Source: CAD feature listing. Evaluate the final solid. Frame: model axes, mm. Face numbers are marked on the shaded views. A direction names the side the tool comes from. Round coordinates to 2 decimals unless told otherwise and drop trailing zeros. Order: outer loops, then holes, each group sorted by start corner. A loop starts at its lowest first (then second) coordinate and runs counter-clockwise, first axis right, second up. Notation, with made-up numbers: (87.5, 4.25) - (123.5, 4.25) arc R34 cw to (123.5, 40.25) - close; hole circle Ø3 at (-38, 86). An arc over 180 degrees is marked (long way). Use one line per item in the form item = value. Start each with the question number.
Q1. Pin query (flat end, axial travel): pin 1 Ø7.5 at (y, z) = (41, 9) entering from +X; pin 2 Ø10.5 at (x, z) = (-64, 9) entering from -Y; pin 3 Ø2 at (x, z) = (109.5, 12) entering from +Y; pin 4 Ø1.5 at (x, y) = (88.5, 2.5) entering from +Z. Return the tip coordinate at first contact, or that it passes through.
Q2. Draft query along Y for the marked faces 1, 2 and 3. Return one class per face: released by +Y, released by -Y, zero draft, split by the parting line, or undercut.
Q3. Cut plane D-D, the plane y = 100.5. Return the cut outline in (x, z).
Q4. Set-up query: the marked faces 4, 5 and 6. Return all of +Z, -Z, +X, -X, +Y, -Y with unobstructed straight access to the full face (end or side cutting, diameter ignored); none if empty.
Q5. Ray query, line 1 (X direction, y = 28, z = 18.25); line 2 (Y direction, x = 24, z = 10); line 3 (X direction, y = -69, z = 5). Return the intervals inside material, ascending. Write a range as [from, to].
Q6. Cut plane B-B, the plane x = 25.5. Return the cut outline in (y, z), and give its area (3 significant figures).
Q7. Cut plane C-C, the plane y = 39. Return the cut outline in (x, z).
Q8. Cut plane A-A, the plane z = 5.5. Return the cut outline in (x, y).
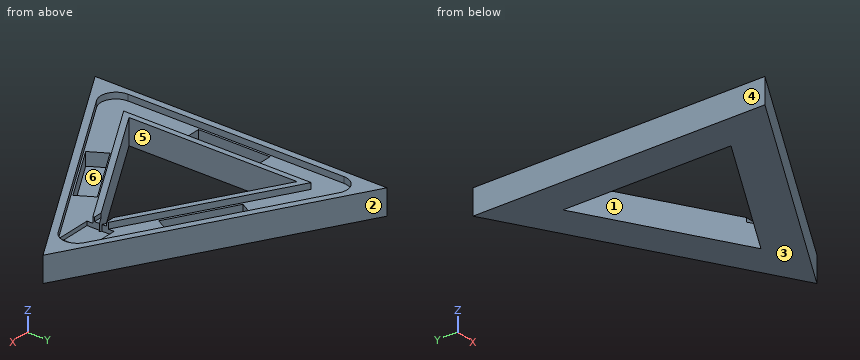
from build123d import *

# Parameters (mm, degrees)
PRISM003_DEPTH         = 6
PRISM002_DEPTH         = 6
BOX004_W               = 10
BOX004_H               = 12
BOX004_DEPTH           = 4
BOX003_W               = 35
BOX003_H               = 26.5
BOX003_DEPTH           = 10
BOX002_W               = 70
BOX002_H               = 19
BOX002_DEPTH           = 19
BOX002_PLACEMENT_ANGLE = 30
BOX001_W               = 70
BOX001_H               = 19
BOX001_DEPTH           = 19
BOX001_PLACEMENT_ANGLE = 90
BOX_W                  = 70
BOX_H                  = 19
BOX_DEPTH              = 19
BOX_PLACEMENT_ANGLE    = 30
PRISM001_DEPTH         = 25
PRISM_DEPTH            = 25
FILLET_R               = 15


with BuildPart() as prism003:
    # Prism003 → Prism003 (new body)
    with BuildSketch(Plane.XY.offset(13)):
        Polygon((106, 0), (-53, 91.798693), (-53, -91.798693), align=None)
    extrude(amount=PRISM003_DEPTH)


with BuildPart() as cut006:
    # Prism002 → Prism002 (new body)
    with BuildSketch(Plane.XY.offset(13)):
        Polygon((152, 0), (-76, 131.635861), (-76, -131.635861), align=None)
    extrude(amount=PRISM002_DEPTH)

    # Cut006: cut Prism003
    add(prism003.part, mode=Mode.SUBTRACT)


with BuildPart() as box004:
    # Box004 → Box004 (new body)
    with BuildSketch(Plane(origin=(84, -6, 15), x_dir=(1, 0, 0), z_dir=(0, 0, 1))):
        with Locations((5, 6)):
            Rectangle(BOX004_W, BOX004_H)
    extrude(amount=BOX004_DEPTH)


with BuildPart() as box003:
    # Box003 → Box003 (new body)
    with BuildSketch(Plane(origin=(93, -13.3, 9), x_dir=(1, 0, 0), z_dir=(0, 0, 1))):
        with Locations((17.5, 13.25)):
            Rectangle(BOX003_W, BOX003_H)
    extrude(amount=BOX003_DEPTH)


with BuildPart() as box002:
    # Box002 → Box002 (new body)
    with BuildSketch(Plane.XY):
        with Locations((35, 9.5)):
            Rectangle(BOX002_W, BOX002_H)
    extrude(amount=BOX002_DEPTH)


with BuildPart() as box002_1:
    # Box002 placement: moved
    add(box002.part.moved(Location((7, -82, 0))).rotate(Axis((7, -82, 0), (0, 0, 1)), BOX002_PLACEMENT_ANGLE))


with BuildPart() as box001:
    # Box001 → Box001 (new body)
    with BuildSketch(Plane.XY):
        with Locations((35, 9.5)):
            Rectangle(BOX001_W, BOX001_H)
    extrude(amount=BOX001_DEPTH)


with BuildPart() as box001_1:
    # Box001 placement: moved
    add(box001.part.moved(Location((-55, -35, 0))).rotate(Axis((-55, -35, 0), (0, 0, 1)), BOX001_PLACEMENT_ANGLE))


with BuildPart() as box:
    # Box → Box (new body)
    with BuildSketch(Plane.XY):
        with Locations((35, 9.5)):
            Rectangle(BOX_W, BOX_H)
    extrude(amount=BOX_DEPTH)


with BuildPart() as box_1:
    # Box placement: moved
    add(box.part.moved(Location((-2, 65, 0))).rotate(Axis((-2, 65, 0), (0, 0, -1)), BOX_PLACEMENT_ANGLE))


with BuildPart() as prism001:
    # Prism001 → Prism001 (new body)
    with BuildSketch(Plane.XY.offset(-6)):
        Polygon((95, 0), (-47.5, 82.272413), (-47.5, -82.272413), align=None)
    extrude(amount=PRISM001_DEPTH)


with BuildPart() as base_fillet:
    # Prism → Prism (new body)
    with BuildSketch(Plane.XY.offset(-6)):
        Polygon((165, 0), (-82.5, 142.894192), (-82.5, -142.894192), align=None)
    extrude(amount=PRISM_DEPTH)

    # Cut: cut Prism001
    add(prism001.part, mode=Mode.SUBTRACT)

    # Cut001: cut Box
    add(box_1.part, mode=Mode.SUBTRACT)

    # Cut002: cut Box001
    add(box001_1.part, mode=Mode.SUBTRACT)

    # Cut003: cut Box002
    add(box002_1.part, mode=Mode.SUBTRACT)

    # Cut004: cut Box003
    add(box003.part, mode=Mode.SUBTRACT)

    # Cut005: cut Box004
    add(box004.part, mode=Mode.SUBTRACT)

    # Cut007: cut Cut006
    add(cut006.part, mode=Mode.SUBTRACT)

    # Fillet
    fillet_edges = [base_fillet.edges().sort_by_distance(p)[0] for p in [
        (152, 0, 16),
        (-76, 131.635861, 16),
        (-76, -131.635861, 16),
    ]]
    fillet(fillet_edges, radius=FILLET_R)


solid = base_fillet.part
Completed:
q1.pin_1 = 100.48
q1.pin_2 = -135.24
q1.pin_3 = 32.62
q1.pin_4 = through
q2.face_1 = undercut
q2.face_2 = released by +Y
q2.face_3 = zero draft
q3.outline = (-82.5, -6) - (-9.07, -6) - (-9.07, 19) - (-22.07, 19) - (-22.07, 13) - (-76, 13) - (-76, 19) - (-82.5, 19) - close
q4.face_4 = +Z, -Z, -X, +Y, -Y
q4.face_5 = +Z, -Z
q4.face_6 = +Z
q5.line_1 = [-82.5, -76], [-53, -47.5], [46.5, 57.5], [103.5, 116.5]
q5.line_2 = [-81.41, -72.19], [-50.25, -40.99], [40.99, 49.99], [71.93, 81.41]
q5.line_3 = [-82.5, -47.5], [-24.51, -0.51], [29.52, 45.49]
q6.outline = (-80.54, -6) - (-40.13, -6) - (-40.13, 19) - (-46.48, 19) - (-46.48, 13) - (-49.38, 13) - (-49.38, 0) - (-71.32, 0) - (-71.32, 13) - (-73.03, 13) - (-73.03, 19) - (-80.54, 19) - close; (40.13, -6) - (80.54, -6) - (80.54, 19) - (73.03, 19) - (73.03, 13) - (71.06, 13) - (71.06, 0) - (49.12, 0) - (49.12, 13) - (46.48, 13) - (46.48, 19) - (40.13, 19) - close
q6.area = 1,130 mm2
q7.outline = (-82.5, -6) - (-47.5, -6) - (-47.5, 19) - (-53, 19) - (-53, 13) - (-76, 13) - (-76, 19) - (-82.5, 19) - close; (27.45, -6) - (97.45, -6) - (97.45, 19) - (84.45, 19) - (84.45, 13) - (63.82, 13) - (63.82, 0) - (43.03, 0) - (43.03, 13) - (38.45, 13) - (38.45, 19) - (27.45, 19) - close
q8.outline = (-82.5, -142.89) - (165, 0) - (-82.5, 142.89) - close; hole (-74, -35) - (-55, -35) - (-55, 35) - (-74, 35) - close; hole (-47.5, -82.27) - (95, 0) - (-47.5, 82.27) - close; hole (-2.5, -65.55) - (7, -82) - (67.62, -47) - (58.12, -30.55) - close; hole (-2, 65) - (58.62, 30) - (68.12, 46.45) - (7.5, 81.45) - close
